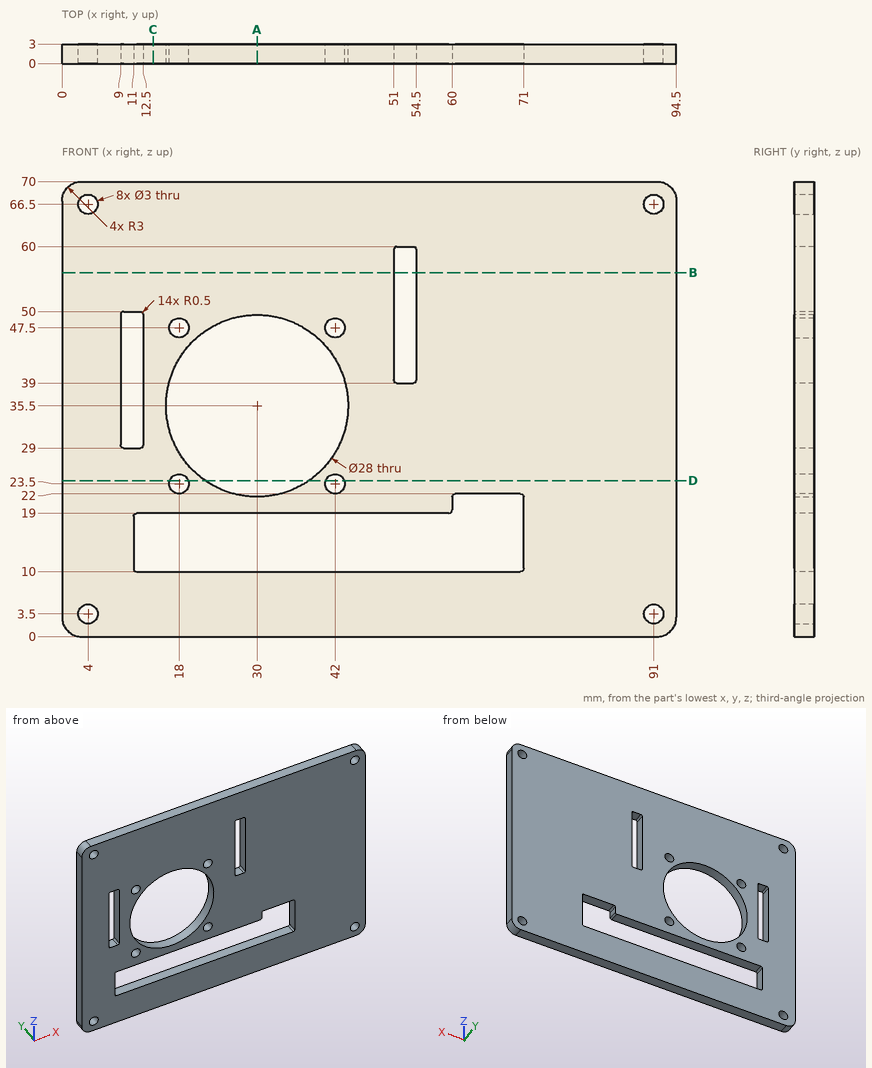
For this review, use the dimensioned drawing (mm, ordinates from the lowest corner) and the shaded views. Coordinates: 2 decimals unless noted, no trailing zeros. Order: outer loops, then holes, each group sorted by start corner. A loop starts at its lowest first (then second) coordinate and runs counter-clockwise, first axis right, second up. Notation, with made-up numbers: M 42,-21 L 77,-21 A29 ccw 77,1 Z; hole C 57,36 d2. An arc over 180 degrees is marked long. Answer as a JSON object with one key per item and string values. Group by question number.
1) For pin 1 (2.5 mm diameter, centred on x = 18, z = 47.5, fed in from +Y), flat-tipped, find the tip position at first contact; note if it passes through.
2) Add section C-C, the plane x = 14. Write out the cut boundary in (y, z).
3) Wall thickness on L1, parallel to X at y = 1.35, z = 35; L2, parallel to Z at x = 91, y = 1.95; L3, parallel to Z at x = 54, y = 2.5: over which ranges is each line inside the solid? List them lowest first.
4) Add section D-D, the plane z = 24. Write out the cut boundary in (x, y).
5) Add section B-B, the plane z = 56. Write out the cut boundary in (x, y).
6) Add section A-A, the plane x = 30. Write out the cut boundary in (y, z).
Computed values:
{
 "1": {"pin 1": "passes through"},
 "2": {"outline": "M 0,0 L 3,0 L 3,10 L 0,10 Z; M 0,19 L 3,19 L 3,70 L 0,70 Z"},
 "3": {"L1": "x = 0 to 9, 12.5 to 16.01, 43.99 to 94.5", "L2": "z = 0 to 2, 5 to 65, 68 to 70", "L3": "z = 0 to 10, 19 to 39, 60 to 70"},
 "4": {"outline": "M 0,0 L 16.59,0 L 16.59,3 L 0,3 Z; M 19.41,0 L 22.02,0 L 22.02,3 L 19.41,3 Z; M 37.98,0 L 40.59,0 L 40.59,3 L 37.98,3 Z; M 43.41,0 L 94.5,0 L 94.5,3 L 43.41,3 Z"},
 "5": {"outline": "M 0,0 L 51,0 L 51,3 L 0,3 Z; M 54.5,0 L 94.5,0 L 94.5,3 L 54.5,3 Z"},
 "6": {"outline": "M 0,0 L 3,0 L 3,10 L 0,10 Z; M 0,19 L 3,19 L 3,21.5 L 0,21.5 Z; M 0,49.5 L 3,49.5 L 3,70 L 0,70 Z"}
}
